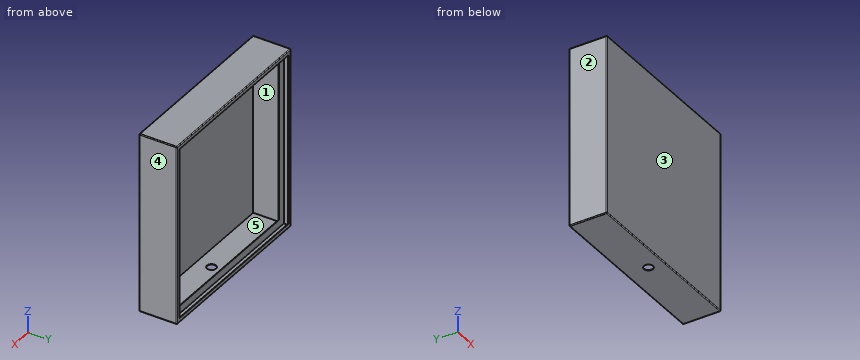
Autodesk Inventor part; units mm, degrees
ref_plane "Work Plane1" through (0, -25.4, 0) normal (0, 1, 0) x (1, 0, 0)
ref_plane "YZ Plane" through (0, 0, 0) normal (1, 0, 0) x (0, 1, 0)
ref_plane "XZ Plane" through (0, 0, 0) normal (0, 1, 0) x (-1, 0, 0)
sketch "Sketch1" plane through (0, 0, 0) normal (0, 1, 0) x (-1, 0, 0)
  line L0 (-462.2267, 0) -> (462.2267, 0)
  line L1 (0, -462.2267) -> (0, 462.2267)
  line L2 (-330.1619, 330.1619) -> (330.1619, 330.1619)
  line L3 (330.1619, 330.1619) -> (330.1619, -330.1619)
  line L4 (330.1619, -330.1619) -> (-330.1619, -330.1619)
  line L5 (-330.1619, -330.1619) -> (-330.1619, 330.1619)
  line L6 (462.2267, 0) -> (-462.2267, 0)
  line L7 (0, -462.2267) -> (0, 462.2267)
  line L8 (314.2869, -314.2869) -> (-314.2869, -314.2869)
  line L9 (-314.2869, -314.2869) -> (-314.2869, 314.2869)
  line L10 (-314.2869, 314.2869) -> (314.2869, 314.2869)
  line L11 (314.2869, 314.2869) -> (314.2869, -314.2869)
  point P0 (0, 0)
  dimension "d0" = 660.3238
  dimension "d2" = 660.3238
  dimension "d123" = 15.875
  dimension "d124" = 15.875
extrude "Extrusion1" add sketch "Sketch1" against normal blind 1.5875 contours L5 L2 L1 L10 L9 L0 | L0 L9 L8 L1 L4 L5 | L1 L8 L11 L0 L3 L4 | L2 L3 L0 L11 L10 L1
sketch "Sketch2" plane through (0, -1.5875, 0) normal (0, -1, 0) x (1, 0, 0)
  line L0 (330.1619, 330.1619) -> (-330.1619, 330.1619)
  line L1 (-330.1619, 330.1619) -> (-330.1619, -330.1619)
  line L2 (-330.1619, -330.1619) -> (330.1619, -330.1619)
  line L3 (330.1619, -330.1619) -> (330.1619, 330.1619)
  line L4 (-314.2869, -314.2869) -> (-314.2869, 314.2869)
  line L5 (-314.2869, 314.2869) -> (314.2869, 314.2869)
  line L6 (314.2869, 314.2869) -> (314.2869, -314.2869)
  line L7 (314.2869, -314.2869) -> (-314.2869, -314.2869)
  line L8 (330.1619, 330.1619) -> (-330.1619, 330.1619)
  line L9 (-330.1619, 330.1619) -> (-330.1619, -330.1619)
  line L10 (-330.1619, -330.1619) -> (330.1619, -330.1619)
  line L11 (330.1619, -330.1619) -> (330.1619, 330.1619)
  line L12 (0, -462.2267) -> (0, 462.2267)
  line L13 (-462.2267, 0) -> (462.2267, 0)
  line L14 (-328.5744, 328.5744) -> (328.5744, 328.5744)
  line L15 (328.5744, 328.5744) -> (328.5744, -328.5744)
  line L16 (328.5744, -328.5744) -> (-328.5744, -328.5744)
  line L17 (-328.5744, -328.5744) -> (-328.5744, 328.5744)
  point P0 (0, 0)
  dimension "d7" = 1.5875
  dimension "d8" = 1.5875
extrude "Extrusion2" add sketch "Sketch2" along normal blind 136.525 contours L3 L13 L15 L14 L12 L0 | L12 L14 L17 L13 L1 L0 | L3 L2 L12 L16 L15 L13 | L13 L17 L16 L12 L2 L1
sketch "Sketch3" plane through (0, -138.1125, 0) normal (0, -1, 0) x (1, 0, 0)
  line L0 (-462.2267, 0) -> (462.2267, 0)
  line L1 (0, -462.2267) -> (0, 462.2267)
  line L2 (-330.1619, 330.1619) -> (330.1619, 330.1619)
  line L3 (330.1619, 330.1619) -> (330.1619, -330.1619)
  line L4 (330.1619, -330.1619) -> (-330.1619, -330.1619)
  line L5 (-330.1619, -330.1619) -> (-330.1619, 330.1619)
  point P0 (0, 0)
extrude "Extrusion3" add sketch "Sketch3" along normal blind 1.5875
ref_plane "Work Plane1" through (0, -25.4, 0) normal (0, 1, 0) x (1, 0, 0)
sketch "Sketch4" plane through (0, -25.4, 0) normal (0, 1, 0) x (1, 0, 0)
  line L0 (328.5744, -328.5744) -> (328.5744, 328.5744)
  line L1 (328.5744, 328.5744) -> (-328.5744, 328.5744)
  line L2 (-328.5744, 328.5744) -> (-328.5744, -328.5744)
  line L3 (-328.5744, -328.5744) -> (328.5744, -328.5744)
  line L4 (-330.1619, -330.1619) -> (-330.1619, 330.1619)
  line L5 (-330.1619, 330.1619) -> (330.1619, 330.1619)
  line L6 (330.1619, 330.1619) -> (330.1619, -330.1619)
  line L7 (330.1619, -330.1619) -> (-330.1619, -330.1619)
  line L8 (-299.9994, 299.9994) -> (299.9994, 299.9994)
  line L9 (299.9994, 299.9994) -> (299.9994, -299.9994)
  line L10 (299.9994, -299.9994) -> (-299.9994, -299.9994)
  line L11 (-299.9994, -299.9994) -> (-299.9994, 299.9994)
  line L12 (462.2267, 0) -> (-462.2267, 0)
  line L13 (0, 462.2267) -> (0, -462.2267)
  point P0 (0, 0)
  dimension "d121" = 30.1625
  dimension "d122" = 30.1625
extrude "Extrusion4" add sketch "Sketch4" against normal blind 1.5875 contours L3 L13 L10 L9 L12 L0 | L12 L9 L8 L13 L1 L0 | L3 L2 L12 L11 L10 L13 | L13 L8 L11 L12 L2 L1
fillet "Fillet1" radius 3.175 12 edges at (0, 0, 330.1619) (0, -139.7, 330.1619) (330.1619, -69.85, 330.1619) (330.1619, -139.7, 0) (330.1619, 0, 0) (330.1619, -69.85, -330.1619) (0, 0, -330.1619) (-330.1619, 0, 0) (-330.1619, -69.85, 330.1619) (0, -139.7, -330.1619) (-330.1619, -69.85, -330.1619) (-330.1619, -139.7, 0)
sketch "Sketch5" plane through (330.1619, 0, -330.1619) normal (0, 0, -1) x (-1, 0, 0)
  line L0 (660.3238, -139.7) -> (0, -139.7)
  line L1 (330.1619, -167.64) -> (330.1619, 27.94)
  circle A0 centre (330.1619, -82.55) radius 16.7005
  line L2 (657.1488, 0) -> (3.175, 0)
  line L3 (3.175, -139.7) -> (657.1488, -139.7)
  point P0 (330.1619, 0)
  dimension "d74" = 57.15
  dimension "d75" = 33.401
extrude "Extrusion10" cut sketch "Sketch5" against normal up to surface (1.5875 mm away)
sketch "Sketch6" plane through (-328.5744, -138.1125, -328.5744) normal (0, 0, 1) x (1, 0, 0)
  circle A0 centre (298.4119, 42.8625) radius 15.875
  circle A1 centre (298.4119, 42.8625) radius 15.875
  circle A2 centre (298.4119, 42.8625) radius 12.7
  point P0 (328.5744, 138.1125)
  dimension "d83" = 25.4
sketch "Sketch7" plane through (330.1619, -136.525, 326.9869) normal (1, 0, 0) x (0, 0, -1)
  line L0 (653.9738, 136.525) -> (0, 136.525)
  line L1 (326.9869, -31.115) -> (326.9869, 164.465)
  circle A0 centre (55.5752, 120.65) radius 3.175
  line L2 (-1.5875, 134.9375) -> (-1.5875, 111.125)
  line L3 (-3.175, 133.35) -> (-3.175, 0)
  circle A1 centre (598.3986, 120.65) radius 3.175
  point P0 (326.9869, 136.525)
  dimension "d91" = 6.35
  dimension "d95" = 58.7502
  dimension "d96" = 15.875
properties part number "Propane Burner" material "Steel"
Source: CAD feature listing. Evaluate the final solid. Frame: model axes, mm. Face numbers are marked on the shaded views. A direction names the side the tool comes from. Coordinates: 2 decimals unless noted, no trailing zeros. Order: outer loops, then holes, each group sorted by start corner. A loop starts at its lowest first (then second) coordinate and runs counter-clockwise, first axis right, second up. Notation, with made-up numbers: M 8,-23.5 L 14,-23.5 A11 ccw 14,-9.5 Z; hole C 25.5,-13.5 d9. An arc over 180 degrees is marked long. Write each question's results on one line, items separated by ' | '. Start each with the question number.
Item 1: Draft query along X for the marked faces 1, 2 and 3. Return one class per face: pulls with the +X half, pulls with the -X half, needs draft (parallel to the pull), parting line crosses it, or undercut.
Item 2: Cut plane C-C (y = -123). Return loops of the section in (x, z) (3 decimals), and give its area (3 significant figures).
Item 3: First-contact query: pin 1 Ø1 at (x, z) = (94.5, -183) entering from +Y; pin 2 Ø1.7 at (y, z) = (-1, -134) entering from +X; pin 3 Ø1.3 at (y, z) = (-0.5, -77) entering from -X. Flat tips, straight axial feed; report the tip coordinate or a pass-through.
Item 4: Line query: probe 1 along Z at (x, y) = (154, -110); probe 2 along Z at (x, y) = (-261, -25.5). Output: solid intervals per line, ascending.
Item 5: Set-up query: the marked faces 4 and 5. Return all of +Z, -Z, +X, -X, +Y, -Y with unobstructed straight access to the full face (end or side cutting, diameter ignored); none if empty.
Checked values:
1) face 1: undercut | face 2: pulls with the -X half | face 3: needs draft
2) outline: M -330.162,-326.987 A3.175 ccw -326.987,-330.162 L 326.987,-330.162 A3.175 ccw 330.162,-326.987 L 330.162,326.987 A3.175 ccw 326.987,330.162 L -326.987,330.162 A3.175 ccw -330.162,326.987 Z; hole M -328.574,-328.574 L 328.574,-328.574 L 328.574,328.574 L -328.574,328.574 Z | area: 4,170 mm2
3) pin 1: stops at y = -138.11 | pin 2: stops at x = 329.87 | pin 3: stops at x = -329.43
4) probe 1: z = -330.16 to -328.57, 328.57 to 330.16 | probe 2: z = -330.16 to -300, 300 to 330.16
5) face 4: +Z, -Z, +X, +Y, -Y | face 5: none
